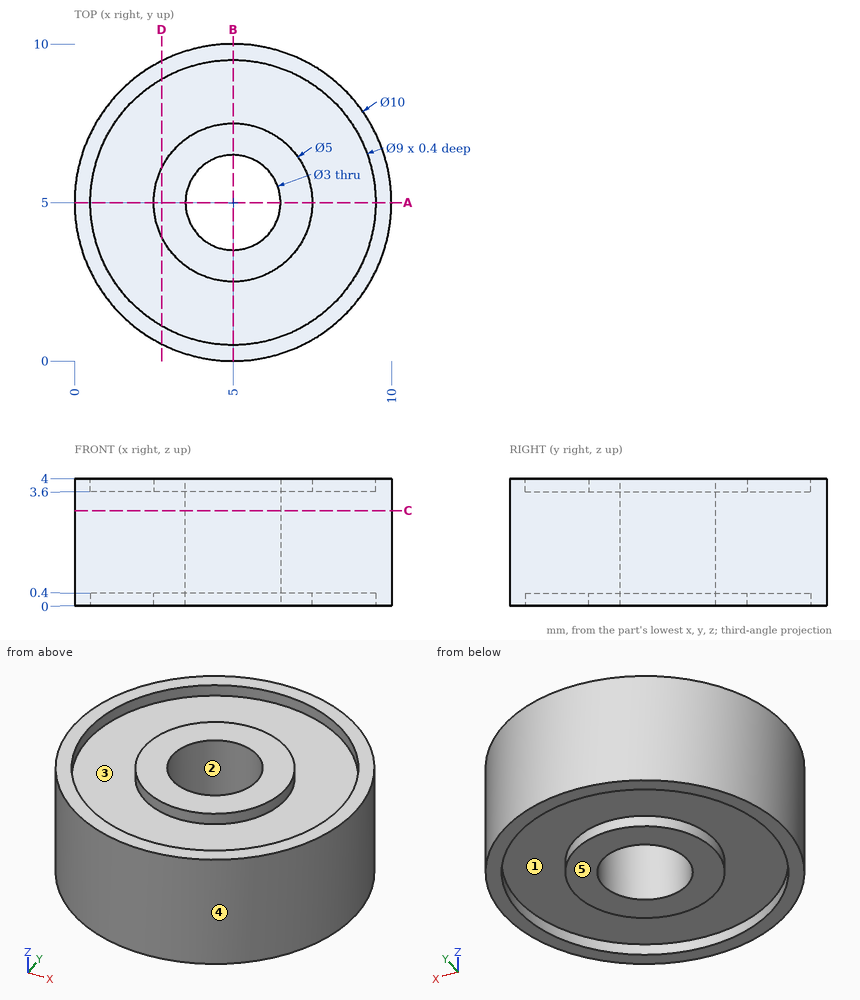
Answer from the drawing. Dimensions are ordinates in mm from the lowest x, y and z of the part. A direction names the side the tool comes from. Coordinates: 2 decimals unless noted, no trailing zeros. Write each loop counter-clockwise with the first axis right and the second up, starting at its lowest first coordinate (ties: lowest second). Pieces come first, ordered by that corner, then holes. Notation, with made-up numbers: M 21.25,0 L 44.25,0 A25 ccw 44.25,26 Z; hole C 51.25,54 d11. An arc over 180 degrees is marked long. Write item = value, one per line.
1. For the marked faces 1 and 2, determine the directions among +Z, -Z, +X, -X, +Y, -Y from which every point of the face is accessible in a straight line to the end or side of a thin tool.
Solution:
face_1 = -Z
face_2 = +Z, -Z
2. Determine the mould class of the marked faces 3, 4 and 5 for opening direction X: released by +X, released by -X, zero draft, split by the parting line, or undercut.
Solution:
face_3 = undercut
face_4 = split by the parting line
face_5 = zero draft
3. A flat-ended cylindrical pin translates along its axis: pin 1 (2 mm diameter, centred on x = 7, z = 3.5, fed in from +Y). Find the tip coordinate at first contact, or state that the pin passes through.
Solution:
pin_1 = 9.9
4. The part is cut by section D-D (x = 2.75). Determine the outline of the cut face in (y, z).
Solution:
outline = M 0.53,0 L 1.1,0 L 1.1,0.4 L 3.91,0.4 L 3.91,0 L 6.09,0 L 6.09,0.4 L 8.9,0.4 L 8.9,0 L 9.47,0 L 9.47,4 L 8.9,4 L 8.9,3.6 L 6.09,3.6 L 6.09,4 L 3.91,4 L 3.91,3.6 L 1.1,3.6 L 1.1,4 L 0.53,4 Z
5. The part is cut by section A-A (y = 5). Determine the outline of the cut face in (x, z).
Solution:
outline = M 0,0 L 0.5,0 L 0.5,0.4 L 2.5,0.4 L 2.5,0 L 3.5,0 L 3.5,4 L 2.5,4 L 2.5,3.6 L 0.5,3.6 L 0.5,4 L 0,4 Z; M 6.5,0 L 7.5,0 L 7.5,0.4 L 9.5,0.4 L 9.5,0 L 10,0 L 10,4 L 9.5,4 L 9.5,3.6 L 7.5,3.6 L 7.5,4 L 6.5,4 Z
6. The part is cut by section C-C (z = 3). Determine the outline of the cut face in (x, y).
Solution:
outline = C 5,5 d10; hole C 5,5 d3
7. Straight lines are drawn through the part: line 1 (Y direction, x = 5, z = 0.1); line 2 (Z direction, x = 1.25, y = 5.25); line 3 (Y direction, x = 5, z = 2.3). For each, find the intervals that lie inside material, in ascending order. Write a range as from..to.
Solution:
line_1 = 0..0.5, 2.5..3.5, 6.5..7.5, 9.5..10
line_2 = 0.4..3.6
line_3 = 0..3.5, 6.5..10
